Read the model definition and answer for the solid it produces. Units are mm, in the model's axes. A direction names the side the tool comes from. Round coordinates to 2 decimals unless told otherwise and drop trailing zeros. Loops run counter-clockwise (first coordinate to the right, second up) from the corner with the lowest first, then second, coordinate; pieces in that order, holes last. Notation, with made-up numbers: (37, -29.5) -> (81, -29.5) arc R17 ccw to (81, 1.5) -> close; hole circle Ø1 at (75.5, 10.25). An arc over 180 degrees is marked (long way). Put each result on its own line as item: value.
from build123d import *

# Parameters (mm, degrees)
SKETCH1_W           = 80
SKETCH1_H           = 30
SKETCH1_W_2         = 77
SKETCH1_H_2         = 27
BOSS_EXTRUDE1_DEPTH = 2
SKETCH1_3_W         = 80
SKETCH1_3_H         = 30
SKETCH1_3_W_2       = 77
SKETCH1_3_H_2       = 27
BOSS_EXTRUDE2_DEPTH = 25
SKETCH2_W           = 25
SKETCH2_H           = 2
BOSS_EXTRUDE3_DEPTH = 23
CUT_EXTRUDE1_DEPTH  = 86.14693183
FILLET1_R           = 1


with BuildPart() as part:
    # Sketch1 → Boss-Extrude1 (new body)
    # profile 1 of 2: a face of its own
    with BuildSketch(Plane(origin=(0, 0, 0), x_dir=(1, 0, 0), z_dir=(0, 1, 0))):
        Rectangle(SKETCH1_W, SKETCH1_H)
        Rectangle(SKETCH1_W_2, SKETCH1_H_2, mode=Mode.SUBTRACT)
    # profile 2 of 2: a face of its own
    with BuildSketch(Plane(origin=(0, 0, 0), x_dir=(1, 0, 0), z_dir=(0, 1, 0))):
        Rectangle(SKETCH1_W_2, SKETCH1_H_2)
    extrude(amount=BOSS_EXTRUDE1_DEPTH)

    # Sketch1<3> → Boss-Extrude2 (add)
    with BuildSketch(Plane(origin=(0, 0, 0), x_dir=(1, 0, 0), z_dir=(0, 1, 0))):
        Rectangle(SKETCH1_3_W, SKETCH1_3_H)
        Rectangle(SKETCH1_3_W_2, SKETCH1_3_H_2, mode=Mode.SUBTRACT)
    extrude(amount=BOSS_EXTRUDE2_DEPTH)

    # Sketch2 → Boss-Extrude3 (add)
    with BuildSketch(Plane(origin=(0, 2, 0), x_dir=(1, 0, 0), z_dir=(0, 1, 0))):
        with Locations((18, 8.6)):
            Rectangle(SKETCH2_W, SKETCH2_H)
        with Locations((18, -8.6)):
            Rectangle(SKETCH2_W, SKETCH2_H)
    extrude(amount=BOSS_EXTRUDE3_DEPTH)

    # Sketch3 → Cut-Extrude1 (cut, through all)
    with BuildSketch(Plane(origin=(40, 0, 0), x_dir=(0, 0, -1), z_dir=(1, 0, 0))):
        with BuildLine():
            Line((-15, 25), (15, 25))
            ThreePointArc((15, 25), (0, 19.270509831), (-15, 25))
        make_face()
    extrude(amount=-CUT_EXTRUDE1_DEPTH, mode=Mode.SUBTRACT)

    # Fillet1
    fillet1_edges = [part.edges().sort_by_distance(p)[0] for p in [
        (-40, 0, 0),
        (0, 0, -15),
        (40, 0, 0),
        (0, 0, 15),
    ]]
    fillet(fillet1_edges, radius=FILLET1_R)


solid = part.part
Item 1: The part is cut by section C-C (z = 0). Determine the outline of the cut face in (x, y).
Derived:
outline: (-40, 1) arc R1 ccw to (-39, 0) -> (39, 0) arc R1 ccw to (40, 1) -> (40, 19.27) -> (38.5, 19.27) -> (38.5, 2) -> (-38.5, 2) -> (-38.5, 19.27) -> (-40, 19.27) -> close
Item 2: Find the intervals of material crossed by line 1 along Z through (x, y) = (14, 16); line 2 along X through (y, z) = (10, -3.5); line 3 along Z through (x, y) = (-27, 17.75), in increasing order.
Derived:
line 1: z = -15 to -13.5, -9.6 to -7.6, 7.6 to 9.6, 13.5 to 15
line 2: x = -40 to -38.5, 38.5 to 40
line 3: z = -15 to -13.5, 13.5 to 15
Item 3: A flat-ended cylindrical pin translates along its axis: pin 1 Ø8 at (x, z) = (-14, -3.5) entering from +Y. Find the tip coordinate at first contact, or state that the pin passes through.
Derived:
pin 1: stops at y = 2
Item 4: The part is cut by section D-D (x = -20). Determine the outline of the cut face in (y, z), then the cut area to 3 significant figures.
Derived:
outline: (0, -14) arc R1 ccw to (1, -15) -> (25, -15) arc R22.5 cw to (23.77, -13.5) -> (2, -13.5) -> (2, 13.5) -> (23.77, 13.5) arc R22.5 cw to (25, 15) -> (1, 15) arc R1 ccw to (0, 14) -> close
area: 127 mm^2
Item 5: Which of the six approach directions +Z, -Z, +X, -X, +Y, -Y give full straight-line access (tool end or side, diameter ignored) to faces 4 (the flat face through (30.5, 12, -9)), 5 (the cylindrical face through (18.18, 20.98, 8.6)), 6 (the flat face through (-1, 13, 15))?
Derived:
face 4: +Y
face 5: +X, -X, +Y
face 6: +Z, +X, -X, +Y, -Y
Item 6: The part is cut by section B-B (x = 12). Determine the outline of the cut face in (y, z).
Derived:
outline: (0, -14) arc R1 ccw to (1, -15) -> (25, -15) arc R22.5 cw to (23.77, -13.5) -> (2, -13.5) -> (2, -9.6) -> (21.42, -9.6) arc R22.5 cw to (20.59, -7.6) -> (2, -7.6) -> (2, 7.6) -> (20.59, 7.6) arc R22.5 cw to (21.42, 9.6) -> (2, 9.6) -> (2, 13.5) -> (23.77, 13.5) arc R22.5 cw to (25, 15) -> (1, 15) arc R1 ccw to (0, 14) -> close
Item 7: For a pull along X with two mould halves and no side action, classify faces 1 (the cylindrical face through (18.175, 20.989, -8.624)), 2 (the flat face through (-1, 13, -13.5)), 3 (the flat face through (40, 10, 0)) as pulls with the +X half, pulls with the -X half, needs draft (parallel to the pull), parting line crosses it, or undercut.
Derived:
face 1: needs draft
face 2: undercut
face 3: pulls with the +X half
Item 8: The part is cut by section A-A (y = 6). Determine the outline of the cut face in (x, z), then the cut area to 3 significant figures.
Derived:
outline: (-40, -15) -> (40, -15) -> (40, 15) -> (-40, 15) -> close; (5.5, -9.6) -> (30.5, -9.6) -> (30.5, -7.6) -> (5.5, -7.6) -> close; (5.5, 7.6) -> (30.5, 7.6) -> (30.5, 9.6) -> (5.5, 9.6) -> close; hole (-38.5, -13.5) -> (38.5, -13.5) -> (38.5, 13.5) -> (-38.5, 13.5) -> close
area: 421 mm^2
